Source: three-view drawing plus pictorial views. Frame: mm from the lowest corner of the part. Round coordinates to 2 decimals unless told otherwise and drop trailing zeros. Loops run counter-clockwise (first coordinate to the right, second up) from the corner with the lowest first, then second, coordinate; pieces in that order, holes last. Notation, with made-up numbers: (11.25, 0) -> (45.25, 0) arc R32 cw to (45.25, 35) -> close; hole circle Ø3 at (69, 54.5). An arc over 180 degrees is marked (long way). Answer in a Markdown table with one row per item. Add a question column.
Q1. Section A-A, the plane y = 38.35. Output: boundary loops of the cut face in (x, z).
Q2. Ray query, L1, parallel to X at y = 46.5, z = 2.6; L2, parallel to Y at x = 35, z = 1.95; L3, parallel to Y at x = 34, z = 0.8. Return the intervals inside material, ascending. Write a range as from..to.
Q3. Section B-B, the plane z = 0.7. Output: boundary loops of the cut face in (x, y) (3 decimals).
Q4. Section D-D, the plane y = 62.5. Output: boundary loops of the cut face in (x, z).
Q5. Section C-C, the plane x = 35. Output: boundary loops of the cut face in (y, z), and give its area (3 significant figures).
Q6. Pin query (flat end, axial travel): pin 1 (2.5 mm diameter, centred on x = 35, y = 62.5, fed in from +Z); pin 2 (6.5 mm diameter, centred on x = 10, y = 38.35, fed in from -Z); pin 3 (0.9 mm diameter, centred on x = 10, z = 1, fed in from -Y); pin 4 (0.9 mm diameter, centred on x = 35.5, z = 1.5, fed in from +Y). Return the tip coordinate at first contact, or that it passes through.
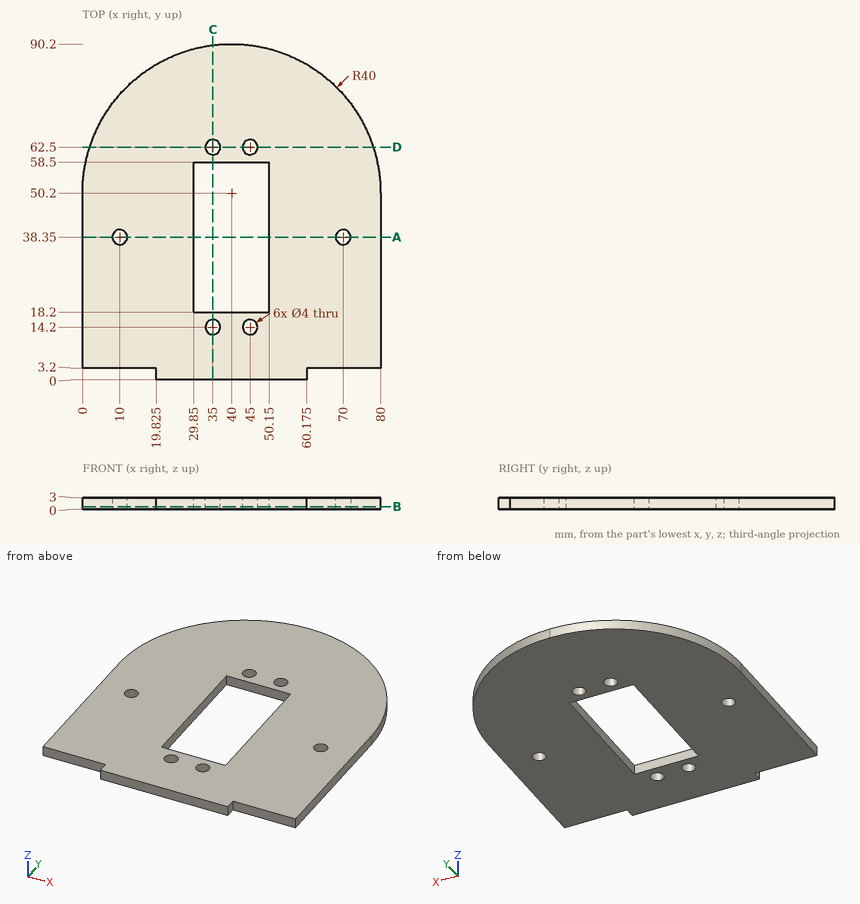
Answer block:
| question | item | result |
|---|---|---|
| 1 | outline | (0, 0) -> (8, 0) -> (8, 3) -> (0, 3) -> close; (12, 0) -> (29.85, 0) -> (29.85, 3) -> (12, 3) -> close; (50.15, 0) -> (68, 0) -> (68, 3) -> (50.15, 3) -> close; (72, 0) -> (80, 0) -> (80, 3) -> (72, 3) -> close |
| 2 | L1 | 0..29.85, 50.15..80 |
| 2 | L2 | 0..12.2, 16.2..18.2, 58.5..60.5, 64.5..89.89 |
| 2 | L3 | 0..12.47, 15.93..18.2, 58.5..60.77, 64.23..89.75 |
| 3 | outline | (0, 3.2) -> (19.825, 3.2) -> (19.825, 0) -> (60.175, 0) -> (60.175, 3.2) -> (80, 3.2) -> (80, 50.2) arc R40 ccw to (0, 50.2) -> close; hole circle Ø4 at (10, 38.35); hole (29.85, 18.2) -> (50.15, 18.2) -> (50.15, 58.5) -> (29.85, 58.5) -> close; hole circle Ø4 at (35, 14.2); hole circle Ø4 at (35, 62.5); hole circle Ø4 at (45, 14.2); hole circle Ø4 at (45, 62.5); hole circle Ø4 at (70, 38.35) |
| 4 | outline | (1.94, 0) -> (33, 0) -> (33, 3) -> (1.94, 3) -> close; (37, 0) -> (43, 0) -> (43, 3) -> (37, 3) -> close; (47, 0) -> (78.06, 0) -> (78.06, 3) -> (47, 3) -> close |
| 5 | outline | (0, 0) -> (12.2, 0) -> (12.2, 3) -> (0, 3) -> close; (16.2, 0) -> (18.2, 0) -> (18.2, 3) -> (16.2, 3) -> close; (58.5, 0) -> (60.5, 0) -> (60.5, 3) -> (58.5, 3) -> close; (64.5, 0) -> (89.89, 0) -> (89.89, 3) -> (64.5, 3) -> close |
| 5 | area | 125 mm^2 |
| 6 | pin 1 | through |
| 6 | pin 2 | z = 0 |
| 6 | pin 3 | y = 3.2 |
| 6 | pin 4 | y = 89.99 |
